```python
from build123d import *

# Parameters (mm, degrees)
SKETCH1_W                                        = 11
SKETCH1_H                                        = 2
SKETCH2_R                                        = 4.4
BOSS_EXTRUDE1_DEPTH                              = 4.2
F_3_5_3_5_DIAMETER_HOLE1_D                       = 3.5
F_3_5_3_5_DIAMETER_HOLE1_DEPTH                   = 2
CBORE_FOR_M3_HEX_HEAD_MACHINE_SCREW1_D           = 3.5
CBORE_FOR_M3_HEX_HEAD_MACHINE_SCREW1_DEPTH       = 6.2
CBORE_FOR_M3_HEX_HEAD_MACHINE_SCREW1_CBORE_D     = 5.7
CBORE_FOR_M3_HEX_HEAD_MACHINE_SCREW1_CBORE_DEPTH = 3


with BuildPart() as part:
    # Sketch1 → Revolve1 (revolve)
    with BuildSketch(Plane(origin=(0, 0, 0), x_dir=(-1, 0, 0), z_dir=(0, 0, -1))):
        with Locations((-5.5, 1)):
            Rectangle(SKETCH1_W, SKETCH1_H)
    revolve(axis=Axis((0, 0, 0), (0, 1, 0)))

    # Sketch2 → Boss-Extrude1 (add)
    with BuildSketch(Plane.XZ):
        Circle(SKETCH2_R)
    extrude(amount=BOSS_EXTRUDE1_DEPTH)

    # Ø3.5 (3.5) Diameter Hole1
    with Locations(Plane(origin=(0, 0, 0), x_dir=(-1, 0, 0), z_dir=(0, -1, 0))):
        with Locations((-8, 0), (0, -8), (8, 0), (0, 8)):
            Hole(F_3_5_3_5_DIAMETER_HOLE1_D / 2, depth=F_3_5_3_5_DIAMETER_HOLE1_DEPTH)

    # CBORE for M3 Hex Head Machine Screw1
    with Locations(Plane(origin=(0, -4.2, 0), x_dir=(-1, 0, 0), z_dir=(0, -1, 0))):
        with Locations((0, 0)):
            CounterBoreHole(CBORE_FOR_M3_HEX_HEAD_MACHINE_SCREW1_D / 2, CBORE_FOR_M3_HEX_HEAD_MACHINE_SCREW1_CBORE_D / 2, CBORE_FOR_M3_HEX_HEAD_MACHINE_SCREW1_CBORE_DEPTH, depth=CBORE_FOR_M3_HEX_HEAD_MACHINE_SCREW1_DEPTH)


solid = part.part
```
Geometry check sheet. Reference: the model listing, model coordinates, mm. A direction names the side the tool comes from. Coordinates: 2 decimals unless noted, no trailing zeros. Loops run counter-clockwise (first coordinate to the right, second up) from the corner with the lowest first, then second, coordinate; pieces in that order, holes last. Notation, with made-up numbers: (27.5, -9.5) - (69.5, -9.5) arc R26 cw to (69.5, 26.5) - close; hole circle Ø8 at (16, -9.5). An arc over 180 degrees is marked (long way). One line per item, written item: value. Start each with the question number.
(1) Tool access check on faces 1 (the cylindrical face through (9.669, 1.014, -0.526)), 2 (the flat face through (0, -1.2, 2)). Record the directions out of +Z, -Z, +X, -X, +Y, -Y that give a thin tool (end or side, any length) a straight path to the whole face; none if there is none.
(2) Cross-section at D-D on y = 1.5. Enter the section's corners in (x, z).
(3) Mould release check, pull along Z, two halves, no side actions. Record for faces 3 (the cylindrical face through (4.197, -2.071, 1.322)), 4 (the flat face through (1, -4.2, -3)), 5 (the cylindrical face through (2.262, -2.721, 1.734)): released by +Z, released by -Z, zero draft, split by the parting line, or undercut.
(4) Material ranges on line 1 (Z direction, x = 0, y = 1); line 2 (X direction, y = 0.5, z = 1.25); line 3 (Z direction, x = 8, y = 1), recorded low to high. Write a range as [from, to].
(5) Depth check by flat-ended pin: P1, Ø8, axis at x = 8, z = 8.5, coming from the -Y side; P2, Ø4, axis at x = 0, z = 0, coming from the -Y side; P3, Ø1.5, axis at x = -0.5, y = -2, coming from the -Z side. Enter the tip coordinate at first touch or a pass-through.
(6) Cross-section at C-C on x = -8. Enter the section's corners in (y, z).
(7) Cross-section at A-A on x = 0. Enter the section's corners in (y, z).
(8) Cross-section at B-B on z = 0. Enter the section's corners in (x, y), plus the area to 3 significant figures.
Results below:
1. face 1: +Y, -Y
1. face 2: -Y
2. outline: circle Ø22 at (0, 0); hole circle Ø3.5 at (-8, 0); hole circle Ø3.5 at (0, -8); hole circle Ø3.5 at (0, 0); hole circle Ø3.5 at (0, 8); hole circle Ø3.5 at (8, 0)
3. face 3: split by the parting line
3. face 4: zero draft
3. face 5: undercut
4. line 1: z = [-11, -9.75], [-6.25, -1.75], [1.75, 6.25], [9.75, 11]
4. line 2: x = [-10.93, -9.22], [-6.78, -1.22], [1.22, 6.78], [9.22, 10.93]
4. line 3: z = [-7.55, -1.75], [1.75, 7.55]
5. P1: stops at y = 0
5. P2: stops at y = -1.2
5. P3: stops at z = -4.4
6. outline: (0, -7.55) - (2, -7.55) - (2, -1.75) - (0, -1.75) - close; (0, 1.75) - (2, 1.75) - (2, 7.55) - (0, 7.55) - close
7. outline: (-4.2, -4.4) - (0, -4.4) - (0, -6.25) - (2, -6.25) - (2, -1.75) - (-1.2, -1.75) - (-1.2, -2.85) - (-4.2, -2.85) - close; (-4.2, 2.85) - (-1.2, 2.85) - (-1.2, 1.75) - (2, 1.75) - (2, 6.25) - (0, 6.25) - (0, 4.4) - (-4.2, 4.4) - close; (0, -11) - (2, -11) - (2, -9.75) - (0, -9.75) - close; (0, 9.75) - (2, 9.75) - (2, 11) - (0, 11) - close
8. outline: (-11, 0) - (-9.75, 0) - (-9.75, 2) - (-11, 2) - close; (-6.25, 0) - (-4.4, 0) - (-4.4, -4.2) - (-2.85, -4.2) - (-2.85, -1.2) - (-1.75, -1.2) - (-1.75, 2) - (-6.25, 2) - close; (1.75, -1.2) - (2.85, -1.2) - (2.85, -4.2) - (4.4, -4.2) - (4.4, 0) - (6.25, 0) - (6.25, 2) - (1.75, 2) - close; (9.75, 0) - (11, 0) - (11, 2) - (9.75, 2) - close
8. area: 38.7 mm2
